Check sheet for the drawn part. Datum: minimum x, y, z corner. Units: mm. A direction names the side the tool comes from. Give positions to 0.01 mm unless a question says otherwise; leave off trailing zeros. Write each loop counter-clockwise with the first axis right and the second up, starting at its lowest first coordinate (ties: lowest second). Pieces come first, ordered by that corner, then holes. Notation, with made-up numbers: (-27, 68.25) -> (20, 68.25) arc R31 ccw to (20, 97.25) -> close; hole circle Ø1 at (49, 49). An arc over 180 degrees is marked (long way). Answer as CSV lines item,"result". Start each with the question number.
1) Tool access check on the marked faces 1 and 2. Record the directions out of +Z, -Z, +X, -X, +Y, -Y that give a thin tool (end or side, any length) a straight path to the whole face; none if there is none.
2) Sectioned sample at D-D on x = 15.75. Record the cut outline in (y, z).
3) Sectioned sample at A-A on z = 11.5. Record the cut outline in (x, y), and give its area (3 significant figures).
4) Sectioned sample at C-C on y = 4.5. Record the cut outline in (x, z), and give its area (3 significant figures).
5) Gauge pin test, flat ends, axial feed: pin 1 Ø1.5 at (y, z) = (6.5, 11.5) entering from +X; pin 2 Ø8 at (x, z) = (12, 20) entering from +Y. Record the tip position at first contact, or that the pin passes through.
6) Sectioned sample at B-B on x = 10. Record the cut outline in (y, z).
7) Material ranges on L1, parallel to X at y = 6.5, z = 11.5; L2, parallel to X at y = 2.1, z = 11.5; L3, parallel to Y at x = 14.25, z = 7, recorded low to high.
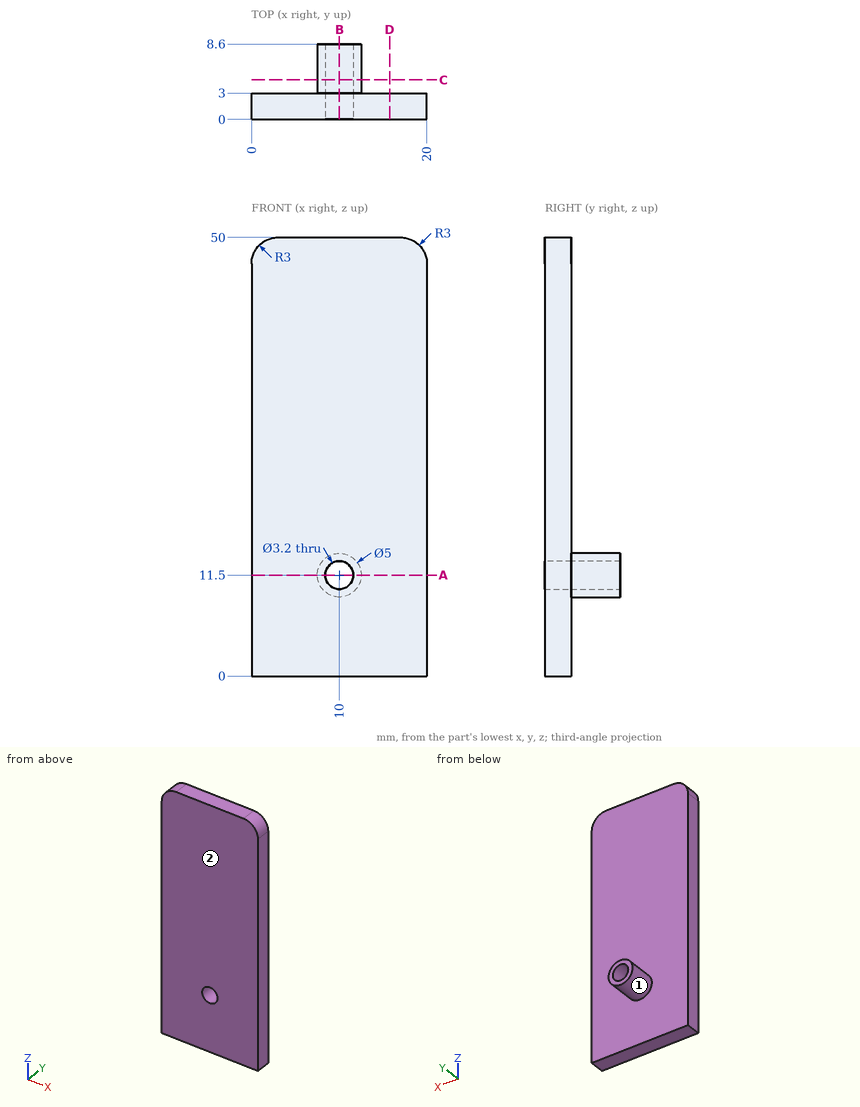
Ans:
1,face 1,"+Y"
1,face 2,"+Z, -Z, +X, -X, -Y"
2,outline,"(0, 0) -> (3, 0) -> (3, 50) -> (0, 50) -> close"
3,outline,"(0, 0) -> (8.4, 0) -> (8.4, 8.6) -> (7.5, 8.6) -> (7.5, 3) -> (0, 3) -> close; (11.6, 0) -> (20, 0) -> (20, 3) -> (12.5, 3) -> (12.5, 8.6) -> (11.6, 8.6) -> close"
3,area,"60.5 mm²"
4,outline,"circle Ø5 at (10, 11.5); hole circle Ø3.2 at (10, 11.5)"
4,area,"11.6 mm²"
5,pin 1,"stops at x = 12.5"
5,pin 2,"stops at y = 3"
6,outline,"(0, 0) -> (3, 0) -> (3, 9) -> (8.6, 9) -> (8.6, 9.9) -> (0, 9.9) -> close; (0, 13.1) -> (8.6, 13.1) -> (8.6, 14) -> (3, 14) -> (3, 50) -> (0, 50) -> close"
7,L1,"x = 7.5 to 8.4, 11.6 to 12.5"
7,L2,"x = 0 to 8.4, 11.6 to 20"
7,L3,"y = 0 to 3"
